Could you check a few things on this model? Use its own coordinates, in mm. A direction names the side the tool comes from. Coordinates: 2 decimals unless noted, no trailing zeros. Loops run counter-clockwise (first coordinate to the right, second up) from the corner with the lowest first, then second, coordinate; pieces in that order, holes last. Notation, with made-up numbers: M 2.5,6.25 L 9.5,6.25 A22 ccw 9.5,13.25 Z; hole C 67.5,-20 d2. An arc over 180 degrees is marked long. Write each question's results on one line, items separated by ' | '.
```python
from build123d import *

# Parameters (mm, degrees)
BOSS_EXTRUDE1_DEPTH = 50.8
FILLET1_R           = 25.4
SKETCH4_W           = 215.9
SKETCH4_H           = 114.3
CUT_EXTRUDE1_DEPTH  = 6.35
BOSS_EXTRUDE2_DEPTH = 6.35
SKETCH6_W           = 25.4
SKETCH6_H           = 25.4
CUT_EXTRUDE2_DEPTH  = 25.4


with BuildPart() as part:
    # Sketch2 → Boss-Extrude1 (new body)
    with BuildSketch(Plane(origin=(0, 0, 0), x_dir=(1, 0, 0), z_dir=(0, 1, 0))):
        with BuildLine():
            Line((-12.7, 12.7), (-63.5, 12.7))
            ThreePointArc((-63.5, 12.7), (-76.2, 0), (-63.5, -12.7))
            Line((-63.5, -12.7), (63.5, -12.7))
            ThreePointArc((63.5, -12.7), (76.2, 0), (63.5, 12.7))
            Line((63.5, 12.7), (12.7, 12.7))
            Line((12.7, 12.7), (12.7, 38.1))
            Line((12.7, 38.1), (127, 38.1))
            Line((127, 38.1), (127, 190.5))
            Line((127, 190.5), (-127, 190.5))
            Line((-127, 190.5), (-127, 38.1))
            Line((-127, 38.1), (-12.7, 38.1))
            Line((-12.7, 38.1), (-12.7, 12.7))
        make_face()
    extrude(amount=BOSS_EXTRUDE1_DEPTH)

    # Fillet1
    fillet1_edges = [part.edges().sort_by_distance(p)[0] for p in [
        (127, 25.4, -38.1),
        (-127, 25.4, -38.1),
        (-127, 25.4, -190.5),
        (127, 25.4, -190.5),
    ]]
    fillet(fillet1_edges, radius=FILLET1_R)

    # Sketch4 → Cut-Extrude1 (cut)
    with BuildSketch(Plane(origin=(0, 50.8, 0), x_dir=(1, 0, 0), z_dir=(0, 1, 0))):
        with Locations((0, 114.3)):
            Rectangle(SKETCH4_W, SKETCH4_H)
    extrude(amount=-CUT_EXTRUDE1_DEPTH, mode=Mode.SUBTRACT)

    # Sketch5 → Boss-Extrude2 (add)
    with BuildSketch(Plane(origin=(0, 44.45, 0), x_dir=(1, 0, 0), z_dir=(0, 1, 0))):
        Polygon((38.1, 114.3), (-19.05, 147.295567884), (-19.05, 81.304432116), align=None)
    extrude(amount=BOSS_EXTRUDE2_DEPTH)

    # Sketch6 → Cut-Extrude2 (cut)
    with BuildSketch(Plane(origin=(0, 50.8, 0), x_dir=(1, 0, 0), z_dir=(0, 1, 0))):
        with Locations((0, 25.4)):
            Rectangle(SKETCH6_W, SKETCH6_H)
    extrude(amount=-CUT_EXTRUDE2_DEPTH, mode=Mode.SUBTRACT)


solid = part.part
```
(1) If we mould it in two halves opening along X, with no side actions, what happens to faces 1 (the flat face through (-2, 48, -171.45)), 2 (the cylindrical face through (119.36, 25.76, -45.34)), 3 (the flat face through (-127, 25, -115))? For each: released by +X, released by -X, zero draft, split by the parting line, or undercut.
Reported:
face 1: undercut | face 2: released by +X | face 3: released by -X
(2) Imagine slicing it at A-A, the plane x = -31.5. List the corners of the cut face in (y, z) for me.
Reported:
outline: M 0,-190.5 L 50.8,-190.5 L 50.8,-171.45 L 44.45,-171.45 L 44.45,-57.15 L 50.8,-57.15 L 50.8,-38.1 L 0,-38.1 Z; M 0,-12.7 L 50.8,-12.7 L 50.8,12.7 L 0,12.7 Z
(3) Imagine slicing it at C-C, the plane z = -76. List the corners of the cut face in (x, y) for me.
Reported:
outline: M -127,0 L 127,0 L 127,50.8 L 107.95,50.8 L 107.95,44.45 L -107.95,44.45 L -107.95,50.8 L -127,50.8 Z
(4) Imagine slicing it at D-D, the plane y = 4. List the corners of the cut face in (x, z) for me, and give its area (3 significant figures).
Reported:
outline: M -127,-165.1 A25.4 ccw -101.6,-190.5 L 101.6,-190.5 A25.4 ccw 127,-165.1 L 127,-63.5 A25.4 ccw 101.6,-38.1 L 12.7,-38.1 L 12.7,-12.7 L 63.5,-12.7 A12.7 ccw 63.5,12.7 L -63.5,12.7 A12.7 ccw -63.5,-12.7 L -12.7,-12.7 L -12.7,-38.1 L -101.6,-38.1 A25.4 ccw -127,-63.5 Z | area: 42,500 mm2
(5) Imagine slicing it at B-B, the plane y = 30.5. List the corners of the cut face in (x, z) for me, and give its area (3 significant figures).
Reported:
outline: M -127,-165.1 A25.4 ccw -101.6,-190.5 L 101.6,-190.5 A25.4 ccw 127,-165.1 L 127,-63.5 A25.4 ccw 101.6,-38.1 L -101.6,-38.1 A25.4 ccw -127,-63.5 Z; M -63.5,-12.7 L 63.5,-12.7 A12.7 ccw 63.5,12.7 L -63.5,12.7 A12.7 ccw Z | area: 41,900 mm2
(6) Please list where these lines run through material, in increasing order: probe 1 along Z at (x, y) = (45.5, 29); probe 2 along Y at (x, z) = (21, -142.5); probe 3 along X at (y, z) = (22, -34). Write a range as from..to.
Reported:
probe 1: z = -190.5..-38.1, -12.7..12.7 | probe 2: y = 0..44.45 | probe 3: x = -12.7..12.7
(7) Will these pins go through, and if not, where does the flat tip stop? P1, Ø3, axis at x = -38.5, z = -67.5, coming from the +Y side; P2, Ø12.5, axis at x = -1.5, z = -28.5, coming from the +Y side; P3, Ø12.5, axis at y = 14.5, z = -26, coming from the -X side.
Reported:
P1: stops at y = 44.45 | P2: stops at y = 25.4 | P3: stops at x = -12.7
(8) Which directions (+Z, -Z, +X, -X, +Y, -Y) give clear straight access to the entire face, cutting with the end or side of a thin tool? Please do faces 4 (the flat face through (12.7, 13, -25)), 5 (the flat face through (-107.95, 48, -113)), 6 (the flat face through (0, 25.4, -26)), 7 (the flat face through (-12.7, 13, -26)).
Reported:
face 4: +X, +Y, -Y | face 5: +Y | face 6: +X, -X, +Y | face 7: -X, +Y, -Y
